Autodesk Inventor part; units mm, degrees
ref_plane "YZ Plane" through (0, 0, 0) normal (1, 0, 0) x (0, 1, 0)
ref_plane "XZ Plane" through (0, 0, 0) normal (0, 1, 0) x (-1, 0, 0)
ref_plane "XY Plane" through (0, 0, 0) normal (0, 0, 1) x (1, 0, 0)
sketch "Sketch1" plane through (0, 0, 0) normal (0, 0, 1) x (1, 0, 0)
  line L0 (0, 0) -> (200, 0)
  line L1 (200, 0) -> (200, 100)
  line L2 (200, 100) -> (0, 100)
  line L3 (0, 100) -> (0, 0)
  dimension "d0" = 200
  dimension "d1" = 100
extrude "Extrusion1" add sketch "Sketch1" along normal blind 3
sketch "Sketch2" plane through (0, 0, 2) normal (-1, 0, 0) x (0, 0, 1)
  line L0 (1, 0) -> (1, 100)
  line L1 (1, 81.5) -> (5, 81.5)
  arc A0 (5, 73.5) -> (5, 81.5) centre (5, 77.5) ccw
  line L2 (5, 73.5) -> (1, 73.5)
  arc A1 (5, 71.5) -> (5, 83.5) centre (5, 77.5) ccw
  line L3 (5, 83.5) -> (1, 83.5)
  line L4 (5, 71.5) -> (1, 71.5)
  line L5 (1, 28.5) -> (5, 28.5)
  arc A2 (5, 16.5) -> (5, 28.5) centre (5, 22.5) ccw
  line L6 (5, 16.5) -> (1, 16.5)
  line L7 (1, 26.5) -> (5, 26.5)
  arc A3 (5, 18.5) -> (5, 26.5) centre (5, 22.5) ccw
  line L8 (5, 18.5) -> (1, 18.5)
  line L9 (1, 50) -> (8.8605, 50) construction
  line L10 (5, 77.5) -> (5, 22.5) construction
  point P0 (-2, 0)
  point P1 (5, 50)
  dimension "d4" = 8
  dimension "d5" = 2
  dimension "d6" = 2
  dimension "d7" = 8
  dimension "d8" = 55
  dimension "d9" = 4
extrude "Extrusion2" add sketch "Sketch2" against normal blind 10 contours L0 L2 A0 L1 L3 A1 L4 | L0 L8 A3 L7 L5 A2 L6
sketch "Sketch3" plane through (0, 0, 3) normal (0, 0, 1) x (1, 0, 0)
  line L0 (0, 71.5) -> (0, 28.5)
  line L1 (0, 50) -> (200, 50) construction
  line L2 (200, 0) -> (200, 100)
  line L3 (68, 30) -> (28, 30)
  line L4 (28, 30) -> (28, 70)
  line L5 (28, 70) -> (68, 70)
  line L6 (68, 70) -> (68, 30)
  line L7 (68, 30) -> (28, 70) construction
  line L8 (28, 30) -> (68, 70) construction
  line L9 (66, 32) -> (30, 32)
  line L10 (30, 32) -> (30, 68)
  line L11 (30, 68) -> (66, 68)
  line L12 (66, 68) -> (66, 32)
  line L13 (66, 32) -> (30, 68) construction
  line L14 (30, 32) -> (66, 68) construction
  line L15 (30, 68) -> (28, 68)
  line L16 (28, 68) -> (28, 32)
  line L17 (28, 32) -> (30, 32)
  line L18 (30, 32) -> (30, 68)
  line L19 (66, 46.75) -> (68, 46.75)
  line L20 (68, 46.75) -> (68, 53.25)
  line L21 (68, 53.25) -> (66, 53.25)
  line L22 (66, 53.25) -> (66, 46.75)
  point P0 (0, 0)
  point P1 (48, 50)
  point P2 (48, 50)
  point P3 (66, 50)
  dimension "d15" = 36
  dimension "d17" = 36
  dimension "d18" = 2
  dimension "d19" = 2
  dimension "d20" = 28
  dimension "d23" = 6.5
extrude "Extrusion3" add sketch "Sketch3" along normal blind 8 contours L3 L4 L17 L9 L12 L19 L6 | L21 L12 L11 L15 L4 L5 L6
sketch "Sketch4" plane through (0, 0, 3) normal (0, 0, 1) x (1, 0, 0)
  line L0 (0, 71.5) -> (0, 28.5)
  line L1 (200, 0) -> (200, 100)
  line L2 (100, 59) -> (130.2, 59)
  line L3 (130.2, 59) -> (130.2, 34.5)
  line L4 (130.2, 34.5) -> (100, 34.5)
  line L5 (100, 34.5) -> (100, 59)
  line L6 (98, 61) -> (132.2, 61)
  line L7 (132.2, 61) -> (132.2, 32.5)
  line L8 (132.2, 32.5) -> (98, 32.5)
  line L9 (98, 32.5) -> (98, 61)
  line L10 (88, 53.6) -> (98, 53.6) construction
  line L11 (98, 46.4) -> (88, 46.4) construction
  line L12 (88, 46.4) -> (88, 53.6) construction
  line L13 (88, 50) -> (0, 50) construction
  line L14 (68, 53.25) -> (68, 70)
  line L15 (98, 53.6) -> (100, 53.6)
  line L16 (98, 46.4) -> (100, 46.4)
  line L17 (130.2, 53.6) -> (132.2, 53.6)
  line L18 (130.2, 46.4) -> (132.2, 46.4)
  line L19 (105.149, 34.5) -> (105.149, 32.5)
  line L20 (129.3871, 34.5) -> (129.3871, 32.5)
  point P0 (0, 0)
  dimension "d24" = 24.5
  dimension "d25" = 30.2
  dimension "d26" = 2
  dimension "d27" = 2
  dimension "d28" = 2
  dimension "d29" = 2
  dimension "d30" = 7.2
  dimension "d31" = 10
  dimension "d32" = 20
  dimension "d33" = 9
extrude "Extrusion4" add sketch "Sketch4" along normal blind 5 contours L5 L15 L9 L6 L7 L17 L3 L2 | L5 L4 L19 L8 L9 L16 | L18 L7 L8 L20 L4 L3
sketch "Sketch5" plane through (0, 0, 0) normal (-1, 0, 0) x (0, 0, 1)
  line L0 (0, 0) -> (0, 100)
  line L1 (3, 0) -> (3, 100)
  line L2 (0, 0) -> (3, 0)
  line L3 (3, 0) -> (3, 100)
  line L4 (3, 100) -> (0, 100)
  line L5 (0, 100) -> (0, 0)
extrude "Extrusion5" add sketch "Sketch5" along normal blind 38
sketch "Sketch6" plane through (0, 0, 3) normal (0, 0, 1) x (1, 0, 0)
  circle A0 centre (-28, 10) radius 1.6
  circle A1 centre (140, 10) radius 1.6
  circle A2 centre (190, 10) radius 1.6
  circle A3 centre (190, 50) radius 1.6
  circle A4 centre (190, 90) radius 1.6
  circle A5 centre (140, 90) radius 1.6
  circle A6 centre (-28, 90) radius 1.6
  line L0 (-28, 90) -> (190, 90) construction
  line L1 (190, 90) -> (190, 10) construction
  line L2 (190, 10) -> (-28, 10) construction
  line L3 (-28, 10) -> (-28, 90) construction
  line L4 (200, 100) -> (-38, 100)
  line L5 (-38, 0) -> (-38, 100)
  line L6 (200, 0) -> (-38, 0)
  line L7 (200, 0) -> (200, 100)
  line L8 (-38, 50) -> (200, 50) construction
  circle A7 centre (-28, 50) radius 1.6
  line L9 (0, 83.5) -> (0, 71.5)
  line L10 (140, 90) -> (140, 10) construction
  line L11 (40, 80) -> (78.5, 80) construction
  line L12 (78.5, 80) -> (78.5, 20) construction
  line L13 (78.5, 20) -> (40, 20) construction
  line L14 (40, 20) -> (40, 80) construction
  circle A8 centre (40, 80) radius 1.6
  circle A9 centre (78.5, 80) radius 1.6
  circle A10 centre (40, 20) radius 1.6
  circle A11 centre (78.5, 20) radius 1.6
  point P0 (0, 0)
  dimension "d38" = 3.2
  dimension "d41" = 3.2
  dimension "d42" = 3.2
  dimension "d43" = 3.2
  dimension "d44" = 3.2
  dimension "d45" = 3.2
  dimension "d48" = 3.2
  dimension "d49" = 10
  dimension "d50" = 10
  dimension "d51" = 10
  dimension "d52" = 10
  dimension "d53" = 3.2
  dimension "d56" = 50
  dimension "d68" = 60
  dimension "d69" = 3.2
  dimension "d70" = 3.2
  dimension "d71" = 3.2
  dimension "d72" = 3.2
  dimension "d73" = 40
  dimension "d74" = 38.5
extrude "Extrusion6" cut sketch "Sketch6" against normal blind 5 contours A0 | A1 | A2 | A3 | A4 | A5 | A6 | A7 | A8 | A9 | A10 | A11
ref_plane "Work Plane1" through (152.2, 32.5, 3) normal (1, 0, 0) x (0, 0, -1)
sketch "Sketch7" plane through (152.2, 32.5, 3) normal (1, 0, 0) x (0, 0, -1)
  line L0 (0, 13.9) -> (0, 2)
  line L1 (0, 13) -> (-5, 13)
  arc A0 (-5, 22) -> (-5, 13) centre (-5, 17.5) ccw
  line L2 (-5, 22) -> (0, 22)
  line L3 (0, 21.1) -> (0, 28.5)
  arc A1 (-5, 21) -> (-5, 14) centre (-5, 17.5) ccw
  line L4 (-5, 14) -> (0, 14)
  line L5 (-5, 21) -> (0, 21)
  line L6 (0, -32.5) -> (0, 67.5)
  line L7 (0, 13.9) -> (-5, 13.9)
  line L8 (0, 21.1) -> (-5, 21.1)
  line L9 (-5, 13.9) -> (-5, 21.1) construction
  line L10 (-5, 17.5) -> (-5, 17.5) construction
  point P0 (3, -32.5)
  point P1 (0, 0)
  dimension "d63" = 3.5
  dimension "d64" = 4.5
  dimension "d65" = 5
extrude "Extrusion7" add sketch "Sketch7" along normal blind 5 contours L0 L1 A0 L2 L3 L6 L5 A1 L4
sketch "Sketch9" plane through (0, 0, 3) normal (0, 0, 1) x (1, 0, 0)
  line L0 (65.5, 10) -> (78.5, 10) construction
  line L1 (78.5, 10) -> (78.5, 90) construction
  line L2 (78.5, 90) -> (65.5, 90) construction
  line L3 (65.5, 90) -> (65.5, 10) construction
  line L4 (65.5, 10) -> (78.5, 90) construction
  line L5 (78.5, 10) -> (65.5, 90) construction
  line L6 (-38, 100) -> (-38, 0)
  line L7 (-38, 50) -> (72, 50) construction
  circle A0 centre (65.5, 90) radius 1.6
  circle A1 centre (78.5, 90) radius 1.6
  circle A2 centre (65.5, 10) radius 1.6
  circle A3 centre (78.5, 10) radius 1.6
  circle A4 centre (-28, 90) radius 1.6
  line L8 (-28, 90) -> (65.5, 90) construction
  point P0 (0, 0)
  dimension "d91" = 110
  dimension "d92" = 3.2
  dimension "d93" = 3.2
  dimension "d94" = 3.2
  dimension "d95" = 3.2
  dimension "d96" = 13
extrude "Extrusion8" cut sketch "Sketch9" against normal blind 10 contours A0 | A1 | A2 | A3
equation "\"d50\" = d49"
equation "\"d51\" = d49"
equation "\"d52\" = d49"
properties part number "lowerBase"
Input: part model. Units: mm. Frame: model coordinates. A direction names the side the tool comes from. Coordinates: 2 decimals unless noted, no trailing zeros. Write each loop counter-clockwise with the first axis right and the second up, starting at its lowest first coordinate (ties: lowest second). Pieces come first, ordered by that corner, then holes.
1) Set-up query: faces 4 (the cylindrical face through (154.7, 49.9, 12.5)), 5 (the flat face through (5, 16.5, 5)), 6 (the flat face through (155, 46.5, 6)). Return all of +Z, -Z, +X, -X, +Y, -Y with unobstructed straight access to the full face (end or side cutting, diameter ignored); none if empty.
2) Pin query (flat end, axial travel): pin 1 Ø1.5 at (x, z) = (156, 4.5) entering from -Y; pin 2 Ø4.5 at (y, z) = (48, 8) entering from -X; pin 3 Ø3 at (y, z) = (22.5, 7.5) entering from +X; pin 4 Ø2.5 at (y, z) = (41, 6) entering from +X. Return the tip coordinate at first contact, or that it passes through.
3) Section C-C on x = -6.5. Output: boundary loops of the cut face in (y, z).
4) Mould query, pull axis Y, two halves, no side actions, for faces 1 (the flat face through (50.9, 68.5, 11)), 2 (the cylindrical face through (4.9, 22.4, 13)), 3 (the flat face through (48, 30, 7)). Classes: pulls with the +Y half, pulls with the -Y half, needs draft (parallel to the pull), parting line crosses it, or undercut.
5) Section A-A on x = 52.5. Output: boundary loops of the cut face in (y, z).
6) Section B-B on y = 64.5. Output: boundary loops of the cut face in (x, z), and give its area (3 significant figures).
7) Material intervals for line 1 along X through (y, z) = (38, 5.75); line 2 along Y through (x, z) = (65.5, 1); line 3 along Y through (x, z) = (40, 0.9), sorted ascending.
Check result:
1. face 4: +Z, +X
1. face 5: +Z, +X, -X, -Y
1. face 6: +X
2. pin 1: stops at y = 45.5
2. pin 2: stops at x = 66
2. pin 3: passes through
2. pin 4: stops at x = 132.2
3. outline: (0, 0) - (100, 0) - (100, 3) - (0, 3) - close
4. face 1: needs draft
4. face 2: undercut
4. face 3: pulls with the -Y half
5. outline: (0, 0) - (100, 0) - (100, 3) - (70, 3) - (70, 11) - (68, 11) - (68, 3) - (32, 3) - (32, 11) - (30, 11) - (30, 3) - (0, 3) - close
6. outline: (-38, 0) - (200, 0) - (200, 3) - (68, 3) - (68, 11) - (66, 11) - (66, 3) - (-38, 3) - close
6. area: 730 mm2
7. line 1: x = 66 to 68, 98 to 100, 130.2 to 132.2
7. line 2: y = 0 to 8.4, 11.6 to 88.4, 91.6 to 100
7. line 3: y = 0 to 18.4, 21.6 to 78.4, 81.6 to 100
